CAD build for the part. Positions are in the model's coordinates, mm. A direction names the side the tool comes from. Round coordinates to 2 decimals unless told otherwise and drop trailing zeros. Write each loop counter-clockwise with the first axis right and the second up, starting at its lowest first coordinate (ties: lowest second). Pieces come first, ordered by that corner, then holes. Notation, with made-up numbers: (39, 75) -> (75, 75) arc R29 cw to (75, 100) -> close; hole circle Ø9 at (35, 18.5). An arc over 180 degrees is marked (long way). Put each result on its own line as item: value. Start each with the question number.
1. 3-axis set-ups, long thin cutter, end or side, ignore diameter. For faces 5 (the flat face through (-27, 7.5, -16)), 6 (the flat face through (-10, 2, 0)), 7 (the flat face through (-27, 0, -8.25)): which of +Z, -Z, +X, -X, +Y, -Y reach the whole face in a straight line?
2. Flat gauge pins, fed straight in: P1, Ø5, axis at x = -10, y = 0, coming from the -Z side; P2, Ø4, axis at y = 4.5, z = -3, coming from the +X side. Where does each tip first touch, or does it go through?
3. Saw through at B-B on z = -13.5. List the corners of the cut face in (x, y), and give its area (3 significant figures).
4. Saw through at C-C on y = 2.5. List the corners of the cut face in (x, z).
5. Saw through at A-A on z = -5.75. List the corners of the cut face in (x, y).
6. Saw through at D-D on x = -13.5. List the corners of the cut face in (y, z), and give its area (3 significant figures).
7. Drill centre lines: line 1 (Y direction, x = -10, z = 0.85); line 2 (Z direction, x = -12.5, y = -6); line 3 (Y direction, x = -26, z = -33). Where is each one in solid material? Low to high. Write a range as from..to.
8. Pull direction X, two halves, no side cores. Call faces 1 (the flat face through (-28, 0, -8)), 2 (the cylindrical face through (8.4, -0.07, 1.97)), 3 (the cylindrical face through (-11.6, -0.07, 1.97)), 4 (the flat face through (-27, 0, -36.847)): pulls with the +X half, pulls with the -X half, needs draft (parallel to the pull), parting line crosses it, or undercut.
Autodesk Fusion 360 part; units mm, degrees
sketch "Skizze1" plane through (0, 0, 0) normal (0, 0, 1) x (1, 0, 0)
  circle A0 centre (-10, 0) radius 1.6
  circle A1 centre (10, 0) radius 1.6
  line L0 (0, 0) -> (0, 16.8871) construction
  arc A2 (10.3958, -3.9804) -> (10.3958, 3.9804) centre (10, 0) ccw
  line L1 (-28, 7.5) -> (-28, -7.5)
  line L2 (10, 0) -> (-66, 0) construction
  line L3 (-25, 7.5) -> (-25, -7.5)
  line L4 (10.3958, 3.9804) -> (-25, 7.5)
  line L5 (10.3958, -3.9804) -> (-25, -7.5)
  line L6 (-25, -7.5) -> (-28, -7.5)
  line L7 (-25, 7.5) -> (-28, 7.5)
  dimension "d1" = 20
  dimension "d2" = 4
  dimension "d3" = 3.2
  dimension "d4" = 28
  dimension "d18" = 15
  dimension "d19" = 3
extrude "Extrusion1" add sketch "Skizze1" along normal blind 4
sketch "Skizze2" plane through (-28, 0, 0) normal (-1, 0, 0) x (0, 0, 1)
  line L0 (0, 7.5) -> (0, -7.5)
  line L1 (4, -7.5) -> (4, 7.5)
  circle A0 centre (-5.75, 0) radius 1.6
  circle A1 centre (-33.5, 0) radius 1.6
  line L2 (-31, -5.75) -> (-31, 5.75)
  line L3 (-31, 5.75) -> (-8.25, 5.75)
  line L4 (-8.25, 5.75) -> (-8.25, -5.75)
  line L5 (-8.25, -5.75) -> (-31, -5.75)
  line L6 (-36.847, 7.5) -> (-36.847, -7.5)
  line L7 (-36.847, -7.5) -> (4, -7.5)
  line L8 (4, -7.5) -> (4, 7.5)
  line L9 (4, 7.5) -> (-36.847, 7.5)
  line L10 (-33.1, 0) -> (0, 0) construction
  circle A2 centre (-25, 0) radius 1.4142 construction
  line L11 (0, -7.5) -> (4, -7.5)
  line L12 (4, 7.5) -> (0, 7.5)
  dimension "d7" = 3.2
  dimension "d8" = 27.75
  dimension "d9" = 19.25
  dimension "d11" = 2.5
  dimension "d12" = 2.5
  dimension "d15" = 25
  dimension "d16" = 15
  dimension "d17" = 11.5
extrude "Extrusion2" add sketch "Skizze2" against normal blind 3 contours L0 L6 L7 L9
Return value:
1. face 5: +Z, -Z, +X, -X, +Y
1. face 6: -Z, +X, +Y, -Y
1. face 7: +X, -X
2. P1: stops at z = 0
2. P2: stops at x = -25
3. outline: (-28, -7.5) -> (-25, -7.5) -> (-25, -5.75) -> (-28, -5.75) -> close; (-28, 5.75) -> (-25, 5.75) -> (-25, 7.5) -> (-28, 7.5) -> close
3. area: 10.5 mm^2
4. outline: (-28, -36.85) -> (-25, -36.85) -> (-25, -31) -> (-28, -31) -> close; (-28, -8.25) -> (-25, -8.25) -> (-25, 0) -> (13.12, 0) -> (13.12, 4) -> (-28, 4) -> close
5. outline: (-28, -7.5) -> (-25, -7.5) -> (-25, -1.6) -> (-28, -1.6) -> close; (-28, 1.6) -> (-25, 1.6) -> (-25, 7.5) -> (-28, 7.5) -> close
6. outline: (-6.36, 0) -> (6.36, 0) -> (6.36, 4) -> (-6.36, 4) -> close
6. area: 50.9 mm^2
7. line 1: y = -6.01..-1.6, 1.6..6.01
7. line 2: z = 0..4
7. line 3: y = -7.5..-1.52, 1.52..7.5
8. face 1: pulls with the -X half
8. face 2: undercut
8. face 3: undercut
8. face 4: needs draft
